```python
from build123d import *


with BuildPart() as part:
    # Sweep1: sweep along a path in Sketch2
    with BuildLine(Plane.XY) as sweep1_path:
        Line((5.4, 53.729321604), (203.4, 33.829572862))
        ThreePointArc((203.4, 33.829572862), (234, 0), (203.4, -33.829572862))
        Line((203.4, -33.829572862), (5.4, -53.729321604))
        ThreePointArc((5.4, -53.729321604), (-54, 0), (5.4, 53.729321604))
    # Sketch3 → Sweep1 (sweep)
    with BuildSketch(Plane(origin=(5.4, 0, 0), x_dir=(0, 0, -1), z_dir=(1, 0, 0))):
        Polygon((-5.579370292, 54), (6.490629708, 54), (9.954731324, 60), (-9.043471907, 60), align=None)
    sweep(path=sweep1_path.line)


solid = part.part
```
Verification items for the finished model (mm, model axes). A direction names the side the tool comes from. Give positions to 0.01 mm unless a question says otherwise; leave off trailing zeros. Order: outer loops, then holes, each group sorted by start corner. A loop starts at its lowest first (then second) coordinate and runs counter-clockwise, first axis right, second up. Notation, with made-up numbers: M -21.75,14 L 26.25,14 A14 cw 26.25,40 Z; hole C 24.5,58 d6. An arc over 180 degrees is marked long. Answer in a Markdown table with one row per item. Add a question column.
Item 1: Tool access check on faces 1 (the cylindrical face through (234.26, 0.73, -0.54)), 2 (the flat face through (104.862, 46.99, -8.215)), 3 (the flat face through (97.53, 47.27, 7.04)). Record the directions out of +Z, -Z, +X, -X, +Y, -Y that give a thin tool (end or side, any length) a straight path to the whole face; none if there is none.
Item 2: Gauge pin test, flat ends, axial feed: pin 1 (4 mm diameter, centred on x = 157.5, z = -3, fed in from -Y); pin 2 (12 mm diameter, centred on x = 167, y = -32, fed in from -Z); pin 3 (6 mm diameter, centred on x = 83.5, y = -45.5, fed in from -Z). Record the tip position at first contact, or that the pin passes through.
Item 3: Section check A-A, the plane z = -1.5. Enter the section's corners in (x, y).
Item 4: Scan lines: probe 1 along Y at (x, z) = (0, -3); probe 2 along X at (y, z) = (0, 3); probe 3 along Y at (x, z) = (195.5, -5.25). Record each from-to range of solid material in increasing order. Write a range as from..to.
Item 5: Mould release check, pull along X, two halves, no side actions. Record for faces 4 (the cylindrical face through (240.218, 1.455, -0.323)), 5 (the flat face through (103.068, -44.184, -0.371)): released by +X, released by -X, zero draft, split by the parting line, or undercut.
Item 6: Section check B-B, the plane x = 199.5. Enter the section's corners in (y, z), and give its area (3 significant figures).
Filled sheet:
| question | item | result |
|---|---|---|
| 1 | face 1 | +Z, -Z |
| 1 | face 2 | -Z |
| 1 | face 3 | +Z |
| 2 | pin 1 | stops at y = -44.91 |
| 2 | pin 2 | stops at z = -6.65 |
| 2 | pin 3 | stops at z = -7.86 |
| 3 | outline | M 5.4,60 A60.24 ccw long 6.65,-59.87 L 204.65,-39.97 A40.24 ccw 203.4,40.1 Z; hole M 5.4,54 A54.27 ccw long 5.45,-53.99 L 203.45,-34.09 A34.27 ccw 203.4,34.1 Z |
| 4 | probe 1 | y = -60.24..-54.27, 54.27..60.24 |
| 4 | probe 2 | x = -60.24..-54.27, 234.27..240.24 |
| 4 | probe 3 | y = -40.89..-34.89, 34.89..40.89 |
| 5 | face 4 | released by +X |
| 5 | face 5 | undercut |
| 6 | outline | M -40.49,-9.95 L -34.49,-6.49 L -34.49,5.58 L -40.49,9.04 Z; M 34.49,-6.49 L 40.49,-9.95 L 40.49,9.04 L 34.49,5.58 Z |
| 6 | area | 186 mm^2 |
